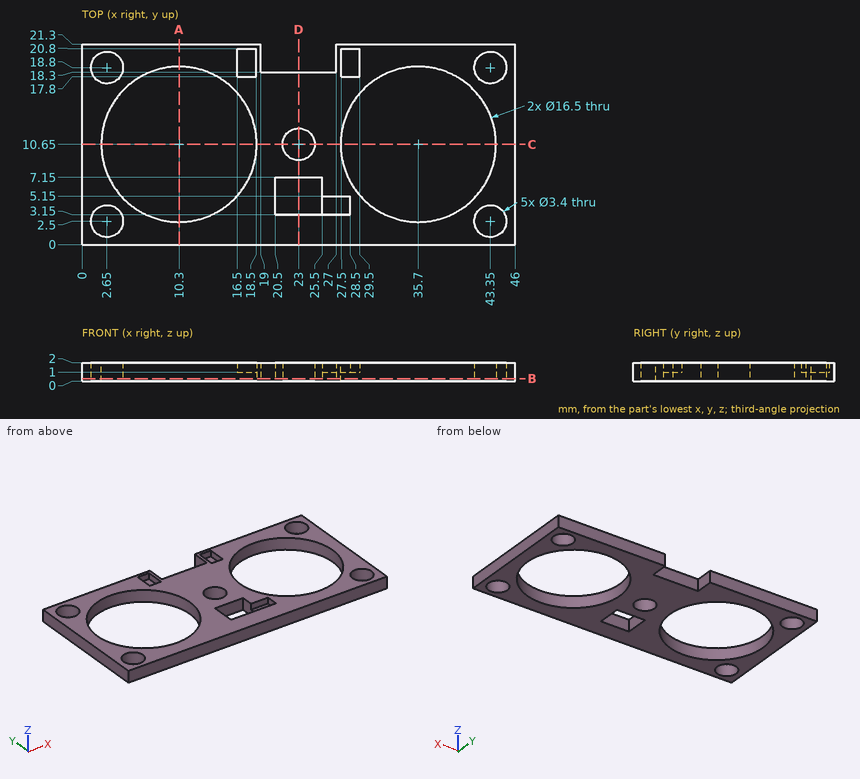
Here's the drawing with two shaded views (mm, measured from the low corner). I have some questions. Round coordinates to 2 decimals unless told otherwise and drop trailing zeros. Loops run counter-clockwise (first coordinate to the right, second up) from the corner with the lowest first, then second, coordinate; pieces in that order, holes last. Notation, with made-up numbers: M 72.5,-24.5 L 99.5,-24.5 A26 cw 99.5,-0.5 Z; hole C 12,70 d4. An arc over 180 degrees is marked long. Put each result on its own line as item: value.
Q1. Imagine slicing it at D-D (x = 23). Write out the boundary of the cut face in (y, z).
Check result:
outline: M 0,0 L 3.15,0 L 3.15,2 L 0,2 Z; M 7.15,0 L 8.95,0 L 8.95,2 L 7.15,2 Z; M 12.35,0 L 18.3,0 L 18.3,2 L 12.35,2 Z
Q2. For pin 1 (0.6 mm diameter, centred on x = 25, z = 1.5, fed in from +Y); pin 2 (1 mm diameter, centred on x = 11, y = 3, fed in from -Z); pin 3 (1.6 mm diameter, centred on x = 17.5, y = 19.5, fed in from +Z), each with a flat end and sliding along its axis, tell me the tip position at first contact or that it passes through.
Check result:
pin 1: y = 18.3
pin 2: through
pin 3: z = 1
Q3. Imagine slicing it at A-A (x = 10.3). Write out the boundary of the cut face in (y, z), then the cut area to 3 significant figures.
Check result:
outline: M 0,0 L 2.4,0 L 2.4,2 L 0,2 Z; M 18.9,0 L 21.3,0 L 21.3,2 L 18.9,2 Z
area: 9.60 mm2
Q4. Imagine slicing it at B-B (z = 0.3). State how many separate pieces and enclosed holes the cut face has, then the cut area to 3 significant figures.
Check result:
separate pieces: 1
enclosed holes: 8
area: 463 mm2
Q5. I need wall thicknesses on probe 1 along X at (y, z) = (10.25, 0.5); probe 2 along Y at (x, z) = (23, 1.45); probe 3 along X at (y, z) = (1, 1.55). Which ranges of each line are inside material? Lowest first, please.
Check result:
probe 1: 0 to 2.06, 18.54 to 21.35, 24.65 to 27.46, 43.94 to 46
probe 2: 0 to 3.15, 7.15 to 8.95, 12.35 to 18.3
probe 3: 0 to 1.85, 3.45 to 42.55, 44.15 to 46
Q6. Imagine slicing it at C-C (y = 10.65). Write out the boundary of the cut face in (x, z), then the cut area to 3 significant figures.
Check result:
outline: M 0,0 L 2.05,0 L 2.05,2 L 0,2 Z; M 18.55,0 L 21.3,0 L 21.3,2 L 18.55,2 Z; M 24.7,0 L 27.45,0 L 27.45,2 L 24.7,2 Z; M 43.95,0 L 46,0 L 46,2 L 43.95,2 Z
area: 19.2 mm2
